from build123d import *

# Parameters (mm, degrees)
SKETCH1_W           = 43.3
SKETCH1_H           = 43.3
SKETCH1_R           = 1.65
BOSS_EXTRUDE1_DEPTH = 1.5
SKETCH2_W           = 23
SKETCH2_H           = 15.7
BOSS_EXTRUDE2_DEPTH = 24.5
SKETCH3_W           = 5.591942039
SKETCH3_H           = 9.785898568
SKETCH3_W_2         = 13.797509161
SKETCH3_H_2         = 6.44288974
BOSS_EXTRUDE3_DEPTH = 7
SKETCH4_R           = 4.168434161
BOSS_EXTRUDE4_DEPTH = 10
SKETCH5_W           = 21
SKETCH5_H           = 5.2
SKETCH5_W_2         = 6.333333334
SKETCH5_H_2         = 15
SKETCH5_W_3         = 6.333333333
CUT_EXTRUDE1_DEPTH  = 24.5


with BuildPart() as part:
    # Sketch1 → Boss-Extrude1 (new body)
    with BuildSketch(Plane(origin=(0, 0, 0), x_dir=(1, 0, 0), z_dir=(0, 1, 0))):
        Rectangle(SKETCH1_W, SKETCH1_H)
        with Locations((-18.35, 18.35)):
            Circle(SKETCH1_R, mode=Mode.SUBTRACT)
        with Locations((18.35, 18.35)):
            Circle(SKETCH1_R, mode=Mode.SUBTRACT)
        with Locations((-18.35, -18.35)):
            Circle(SKETCH1_R, mode=Mode.SUBTRACT)
        with Locations((18.35, -18.35)):
            Circle(SKETCH1_R, mode=Mode.SUBTRACT)
    extrude(amount=BOSS_EXTRUDE1_DEPTH)

    # Sketch2 → Boss-Extrude2 (add)
    with BuildSketch(Plane(origin=(0, 1.5, 0), x_dir=(1, 0, 0), z_dir=(0, 1, 0))):
        with Locations((0, 13.8)):
            Rectangle(SKETCH2_W, SKETCH2_H)
    extrude(amount=BOSS_EXTRUDE2_DEPTH)

    # Sketch3 → Boss-Extrude3 (add)
    with BuildSketch(Plane(origin=(0, 1.5, 0), x_dir=(1, 0, 0), z_dir=(0, 1, 0))):
        with Locations((-18.325766573, -6.44288974)):
            Rectangle(SKETCH3_W, SKETCH3_H)
        with Locations((-7.84087525, -17.353254914)):
            Rectangle(SKETCH3_W_2, SKETCH3_H_2)
    boss_extrude3 = extrude(amount=BOSS_EXTRUDE3_DEPTH)

    # Mirror1: Boss-Extrude3 across plane
    add(boss_extrude3.mirror(Plane(origin=(0, 0, 0), x_dir=(0, 0, 1), z_dir=(1, 0, 0))))

    # Sketch4 → Boss-Extrude4 (add)
    with BuildSketch(Plane(origin=(0, 1.5, 0), x_dir=(1, 0, 0), z_dir=(0, 1, 0))):
        with Locations((-8.592825404, -0.943272563)):
            Circle(SKETCH4_R)
        with Locations((7.765846719, -8.463609984)):
            Circle(SKETCH4_R)
    extrude(amount=BOSS_EXTRUDE4_DEPTH)

    # Sketch5 → Cut-Extrude1 (cut)
    with BuildSketch(Plane(origin=(0, 26, 0), x_dir=(1, 0, 0), z_dir=(0, 1, 0))):
        with Locations((0, 8.55)):
            Rectangle(SKETCH5_W, SKETCH5_H)
        with Locations((0, 21.65)):
            Rectangle(SKETCH5_W_2, SKETCH5_H_2)
        with Locations((7.333333334, 21.65)):
            Rectangle(SKETCH5_W_3, SKETCH5_H_2)
        with Locations((-7.333333334, 21.65)):
            Rectangle(SKETCH5_W_3, SKETCH5_H_2)
    extrude(amount=-CUT_EXTRUDE1_DEPTH, mode=Mode.SUBTRACT)


solid = part.part
Here's how the part is built. I have some questions about the finished solid (model axes, mm). A direction names the side the tool comes from. Round coordinates to 2 decimals unless told otherwise and drop trailing zeros. Write each loop counter-clockwise with the first axis right and the second up, starting at its lowest first coordinate (ties: lowest second). Pieces come first, ordered by that corner, then holes. Notation, with made-up numbers: (87, -12) -> (101, -12) arc R23 cw to (101, 8) -> close; hole circle Ø7 at (86.5, 84). An arc over 180 degrees is marked (long way). One line per item, written item: value.
1) I'm going to push flat-ended pins straight in: pin 1 Ø1.9 at (x, z) = (11, 17) entering from +Y; pin 2 Ø2 at (x, y) = (6, 6.5) entering from -Z; pin 3 Ø5 at (y, z) = (18.5, -12.5) entering from -X; pin 4 Ø6 at (y, z) = (16, 2) entering from +X. Where does each tip first touch, or does it pass through?
Filled sheet:
pin 1: stops at y = 8.5
pin 2: stops at z = -14.15
pin 3: stops at x = -11.5
pin 4: passes through
2) Suppose I cut it at A-A on x = -18.35. List the corners of the cut face in (y, z) for me, plus the area to 3 significant figures.
Filled sheet:
outline: (0, -21.65) -> (1.5, -21.65) -> (1.5, -20) -> (0, -20) -> close; (0, -16.7) -> (1.5, -16.7) -> (1.5, 1.55) -> (8.5, 1.55) -> (8.5, 11.34) -> (1.5, 11.34) -> (1.5, 16.7) -> (0, 16.7) -> close; (0, 20) -> (1.5, 20) -> (1.5, 21.65) -> (0, 21.65) -> close
area: 124 mm2
3) For faces 5 (the face through (8, 5, 20.575)), 6 (the face through (0.942, 5, 17)), 7 (the face through (11.5, 14, -14)), which set-ups out of +Z, -Z, +X, -X, +Y, -Y let a thin tool reach every point of the face, with its end or its side?
Filled sheet:
face 5: +Z, +X, -X, +Y
face 6: +Z, +Y
face 7: -Z, +X, +Y
4) Suppose I cut it at B-B on z = -18.35. List the corners of the cut face in (x, y) for me.
Filled sheet:
outline: (-21.65, 0) -> (-20, 0) -> (-20, 1.5) -> (-21.65, 1.5) -> close; (-16.7, 0) -> (16.7, 0) -> (16.7, 1.5) -> (11.5, 1.5) -> (11.5, 26) -> (10.5, 26) -> (10.5, 1.5) -> (4.17, 1.5) -> (4.17, 26) -> (3.17, 26) -> (3.17, 1.5) -> (-3.17, 1.5) -> (-3.17, 26) -> (-4.17, 26) -> (-4.17, 1.5) -> (-10.5, 1.5) -> (-10.5, 26) -> (-11.5, 26) -> (-11.5, 1.5) -> (-16.7, 1.5) -> close; (20, 0) -> (21.65, 0) -> (21.65, 1.5) -> (20, 1.5) -> close
5) If I drill on line 1 (Z direction, x = -18.35, y = 0.75); line 2 (Z direction, x = 11, y = 5.25), over which ranges is the centre line in solid material (lowest first)? Write a range as [from, to].
Filled sheet:
line 1: z = [-21.65, -20], [-16.7, 16.7], [20, 21.65]
line 2: z = [-21.65, -5.95], [5.83, 11.09], [14.13, 20.57]
6) We'd pull the mould along X, two halves only. Please class faces 1 (the face through (-8, 5, 14.132)), 2 (the face through (10.5, 14, -18)), 3 (the face through (-11.5, 14, -14)), 4 (the face through (-10.5, 14, -9)): released by +X, released by -X, zero draft, split by the parting line, or undercut.
Filled sheet:
face 1: zero draft
face 2: undercut
face 3: released by -X
face 4: undercut
7) Suppose I cut it at C-C on x = 14. List the corners of the cut face in (y, z) for me.
Filled sheet:
outline: (0, -21.65) -> (1.5, -21.65) -> (1.5, 14.13) -> (8.5, 14.13) -> (8.5, 20.57) -> (1.5, 20.57) -> (1.5, 21.65) -> (0, 21.65) -> close
8) Suppose I cut it at D-D on y = 10.5. List the corners of the cut face in (x, z) for me, plus the area to 3 significant figures.
Filled sheet:
outline: circle Ø8.34 at (-8.59, 0.94); (-11.5, -21.65) -> (-10.5, -21.65) -> (-10.5, -14.15) -> (-4.17, -14.15) -> (-4.17, -21.65) -> (-3.17, -21.65) -> (-3.17, -14.15) -> (3.17, -14.15) -> (3.17, -21.65) -> (4.17, -21.65) -> (4.17, -14.15) -> (10.5, -14.15) -> (10.5, -21.65) -> (11.5, -21.65) -> (11.5, -5.95) -> (10.5, -5.95) -> (10.5, -11.15) -> (-10.5, -11.15) -> (-10.5, -5.95) -> (-11.5, -5.95) -> close; circle Ø8.34 at (7.77, 8.46)
area: 219 mm2
